Check sheet for the modelled part. Datum: model origin and axes. Units: mm. Face numbers are marked on the shaded views. Coordinates: 2 decimals unless noted, no trailing zeros. Write each loop counter-clockwise with the first axis right and the second up, starting at its lowest first coordinate (ties: lowest second). Pieces come first, ordered by that corner, then holes. Notation, with made-up numbers: (68.25, 16) -> (124.25, 16) arc R20 cw to (124.25, 40) -> close; hole circle Ø7 at (28, -20). An arc over 180 degrees is marked (long way). Put each result on its own line as item: value.
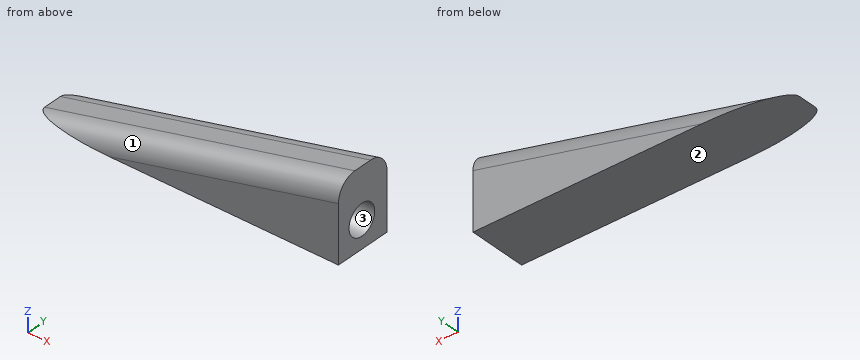
```python
from build123d import *

# Parameters (mm, degrees)
F1_DEPTH = 38.1
F2_R     = 12.877415
F3_R     = 10.088081
F4_DEPTH = 50.8


with BuildPart() as f1:
    # F0 (on Front) → F1 (new body)
    with BuildSketch(Plane.XZ):
        Polygon((-103.93265, 0), (99.26735, 0), (99.26735, 50.8), align=None)
    extrude(amount=F1_DEPTH)

    # F2
    f2_edges = [f1.edges().sort_by_distance(p)[0] for p in [
        (-2.33265, 0, 25.4),
        (-2.33265, -38.1, 25.4),
    ]]
    fillet(f2_edges, radius=F2_R)

    # F3 (on face) → F4 (cut)
    with BuildSketch(Plane.YZ.offset(99.26735)):
        with Locations((-19.710729, 18.024944)):
            Circle(F3_R)
    extrude(amount=-F4_DEPTH, mode=Mode.SUBTRACT)


solid = f1.part
```
Q1. Material ranges on line 1 along Z through (x, y) = (-75.5, -3.5); line 2 along Z through (x, y) = (-18.5, -33.5); line 3 along Z through (x, y) = (80, -21), recorded low to high.
Recorded:
line 1: z = 0 to 2.93
line 2: z = 0 to 18.25
line 3: z = 0 to 8.02, 28.03 to 45.98
Q2. Cross-section at C-C (y = -7). Record the cut outline in (x, z), plus the area to 3 significant figures.
Recorded:
outline: (-98.08, 0) -> (99.27, 0) -> (99.27, 49.34) -> close
area: 4,870 mm2
Q3. Depth check by flat-ended pin: P1, Ø5, axis at x = 49, z = 38.5, coming from the +Y side; P2, Ø6, axis at y = -16, z = 21, coming from the +X side; P3, Ø5, axis at x = -42.5, z = 9, coming from the -Y side; P4, Ø8, axis at x = -3.5, y = -11, coming from the -Z side. Enter the tip coordinate at first touch or a pass-through.
Recorded:
P1: stops at y = -5.62
P2: stops at x = 48.47
P3: stops at y = -37.39
P4: stops at z = 0
Q4. Cross-section at B-B (y = -18.5). Record the cut outline in (x, z).
Recorded:
outline: (-103.93, 0) -> (99.27, 0) -> (99.27, 8.01) -> (48.47, 8.01) -> (48.47, 28.04) -> (99.27, 28.04) -> (99.27, 50.8) -> close
Q5. Mould release check, pull along Z, two halves, no side actions. Record for the marked faces 1, 2 and 3: released by +Z, released by -Z, zero draft, split by the parting line, or undercut.
Recorded:
face 1: released by +Z
face 2: released by -Z
face 3: undercut
Q6. Cross-section at A-A (y = -27). Record the cut outline in (x, z), plus the area to 3 significant figures.
Recorded:
outline: (-103.42, 0) -> (99.27, 0) -> (99.27, 11.05) -> (48.47, 11.05) -> (48.47, 25) -> (99.27, 25) -> (99.27, 50.67) -> close
area: 4,430 mm2
